The listing builds one solid part. Answer for the finished solid, in the listing's coordinates (mm). Round coordinates to 2 decimals unless told otherwise and drop trailing zeros. Write each loop counter-clockwise with the first axis right and the second up, starting at its lowest first coordinate (ties: lowest second). Pieces come first, ordered by that corner, then holes.
Item 1: Find the intervals of material crossed by probe 1 along Y at (x, z) = (-19.05, -6); probe 2 along X at (y, z) = (15, -8.75); probe 3 along Y at (x, z) = (0, -1), in increasing order.
Item 2: This flat-tipped pin is pushed along its axis until it touches: pin 1 (6 mm diameter, centred on x = 19.05, y = 16.256, fed in from -Z). Where does it stop, or does it pass through?
Item 3: Find section C-C on z = 5.25. Give the vertices of the cut face in (x, y), then the cut area to 3 significant figures.
Item 4: For a pull along Y with two mould halves and no side action, classify faces 1 (the face through (15.082, 13.214, -0.178)), 2 (the face through (-1, 37.084, 0)), 3 (the face through (1, -12.224, 0)) as +Y half, -Y half, draft (parallel to the pull), parting line (faces both ways), or undercut.
Item 5: Find section A-A on x = -19.05. Give the vertices of the cut face in (y, z).
Item 6: Find section B-B on y = 0. Give the vertices of the cut face in (x, z), then the cut area to 3 significant figures.
```python
from build123d import *

# Parameters (mm, degrees)
SKETCH1_R           = 5
SKETCH1_R_2         = 8.5
BOSS_EXTRUDE2_DEPTH = 12.7


with BuildPart() as part:
    # Sketch1 → Boss-Extrude2 (new, symmetric)
    with BuildSketch(Plane.XY):
        Polygon((-38.1, 37.084), (38.1, 37.084), (38.1, 12.224), (38.1, -12.224), (-38.1, -12.224), (-38.1, 12.224), align=None)
        with Locations((-19.05, 16.256)):
            Circle(SKETCH1_R, mode=Mode.SUBTRACT)
        with Locations((19.05, 16.256)):
            Circle(SKETCH1_R, mode=Mode.SUBTRACT)
        Circle(SKETCH1_R_2, mode=Mode.SUBTRACT)
    extrude(amount=BOSS_EXTRUDE2_DEPTH, both=True)


solid = part.part
```
Check values:
1. probe 1: y = -12.22 to 11.26, 21.26 to 37.08
1. probe 2: x = -38.1 to -23.89, -14.21 to 14.21, 23.89 to 38.1
1. probe 3: y = -12.22 to -8.5, 8.5 to 37.08
2. pin 1: passes through
3. outline: (-38.1, -12.22) - (38.1, -12.22) - (38.1, 37.08) - (-38.1, 37.08) - close; hole circle Ø10 at (-19.05, 16.26); hole circle Ø17 at (0, 0); hole circle Ø10 at (19.05, 16.26)
3. area: 3,370 mm2
4. face 1: undercut
4. face 2: +Y half
4. face 3: -Y half
5. outline: (-12.22, -12.7) - (11.26, -12.7) - (11.26, 12.7) - (-12.22, 12.7) - close; (21.26, -12.7) - (37.08, -12.7) - (37.08, 12.7) - (21.26, 12.7) - close
6. outline: (-38.1, -12.7) - (-8.5, -12.7) - (-8.5, 12.7) - (-38.1, 12.7) - close; (8.5, -12.7) - (38.1, -12.7) - (38.1, 12.7) - (8.5, 12.7) - close
6. area: 1,500 mm2
